Build history of the part. All positions in model axes, mm. Give positions to 0.01 mm unless a question says otherwise; leave off trailing zeros. Write each loop counter-clockwise with the first axis right and the second up, starting at its lowest first coordinate (ties: lowest second). Pieces come first, ordered by that corner, then holes. Notation, with made-up numbers: (23, 74.5) -> (50, 74.5) arc R33 cw to (50, 108.5) -> close; hole circle Ø7 at (33, -19). An arc over 180 degrees is marked (long way). Write item = value, one per line. Start each with the question number.
Q1. Saw through at C-C, the plane z = 0.3. Give the number of separate pieces and of enclosed holes in the cut face, then the cut area to 3 significant figures.
Q2. Wall check: line 1 (Y direction, x = 35, z = 1); line 2 (Y direction, x = 66, z = 1.05); line 3 (X direction, y = 85, z = 0.6). Give the ranges that are in metal, low to high.
Q3. Saw through at B-B, the plane x = 35. List the corners of the cut face in (y, z), then the cut area to 3 significant figures.
Q4. Saw through at A-A, the plane y = 75. List the corners of the cut face in (x, z).
Q5. Mould opens along X. For faces 1 (the face through (39.87, 121.66, 0.76)), 2 (the face through (40, 81, 0)) say: pulls with the +X half, pulls with the -X half, needs draft (parallel to the pull), parting line crosses it, or undercut.
from build123d import *

# Parameters (mm, degrees)
EXTRUDE_1_DEPTH      = 1.5
CUT_EXTRUDE_1_DEPTH  = 1.5
SKETCH_3_R           = 2
CUT_EXTRUDE_2_DEPTH  = 1.5
SKETCH_4_W           = 80
SKETCH_4_H           = 5
EXTRUDE_2_DEPTH      = 1.5
FILLET_1_R           = 2
SKETCH_5_OUTSIDE_W   = 163.618
SKETCH_5_OUTSIDE_H   = 213.618
SKETCH_5_OUTSIDE_W_2 = 80
SKETCH_5_OUTSIDE_H_2 = 170
CUT_EXTRUDE_3_DEPTH  = 193.943644622
SKETCH_6_R           = 1.5
CUT_EXTRUDE_4_DEPTH  = 184.377343202
SKETCH_7_W           = 6
SKETCH_7_H           = 170
CUT_EXTRUDE_5_DEPTH  = 10
FILLET_2_R           = 2
FILLET_3_R           = 1
FILLET_4_R           = 1


with BuildPart() as part:
    # 草图1 → 凸台-拉伸1 (new body)
    with BuildSketch(Plane.XY):
        Polygon((80, 90), (100, 90), (100, 70), (80, 70), (80, 0), (0, 0), (0, 70), (-20, 70), (-20, 90), (0, 90), (0, 160), (80, 160), align=None)
    extrude(amount=EXTRUDE_1_DEPTH)

    # 草图2 → 切除-拉伸1 (cut)
    with BuildSketch(Plane.XY.offset(1.5)):
        with BuildLine():
            Line((64, 153.5), (80, 153.5))
            Line((80, 153.5), (80, 156.5))
            Line((80, 156.5), (64, 156.5))
            ThreePointArc((64, 156.5), (62.5, 155), (64, 153.5))
        make_face()
        with BuildLine():
            Line((38.5, 5), (38.5, 15))
            ThreePointArc((38.5, 15), (40, 21.66227766), (41.5, 15))
            Line((41.5, 15), (41.5, 5))
            ThreePointArc((41.5, 5), (40, 3.5), (38.5, 5))
        make_face()
        with BuildLine():
            Line((16, 153.5), (0, 153.5))
            Line((0, 153.5), (0, 156.5))
            Line((0, 156.5), (16, 156.5))
            ThreePointArc((16, 156.5), (17.5, 155), (16, 153.5))
        make_face()
        with BuildLine():
            Line((64, 103.5), (80, 103.5))
            Line((80, 103.5), (80, 106.5))
            Line((80, 106.5), (64, 106.5))
            ThreePointArc((64, 106.5), (62.5, 105), (64, 103.5))
        make_face()
        with BuildLine():
            Line((16, 106.5), (0, 106.5))
            Line((0, 106.5), (0, 103.5))
            Line((0, 103.5), (16, 103.5))
            ThreePointArc((16, 103.5), (17.5, 105), (16, 106.5))
        make_face()
        with BuildLine():
            Line((16, 56.5), (0, 56.5))
            Line((0, 56.5), (0, 53.5))
            Line((0, 53.5), (16, 53.5))
            ThreePointArc((16, 53.5), (17.5, 55), (16, 56.5))
        make_face()
        with BuildLine():
            Line((64, 53.5), (80, 53.5))
            Line((80, 53.5), (80, 56.5))
            Line((80, 56.5), (64, 56.5))
            ThreePointArc((64, 56.5), (62.5, 55), (64, 53.5))
        make_face()
        with BuildLine():
            Line((16, 6.5), (0, 6.5))
            Line((0, 6.5), (0, 3.5))
            Line((0, 3.5), (16, 3.5))
            ThreePointArc((16, 3.5), (17.5, 5), (16, 6.5))
        make_face()
        with BuildLine():
            Line((64, 6.5), (80, 6.5))
            Line((80, 6.5), (80, 3.5))
            Line((80, 3.5), (64, 3.5))
            ThreePointArc((64, 3.5), (62.5, 5), (64, 6.5))
        make_face()
        with BuildLine():
            Line((38.5, 155), (38.5, 145))
            ThreePointArc((38.5, 145), (40, 138.33772234), (41.5, 145))
            Line((41.5, 145), (41.5, 155))
            ThreePointArc((41.5, 155), (40, 156.5), (38.5, 155))
        make_face()
        with BuildLine():
            Line((41.5, 55), (41.5, 45))
            ThreePointArc((41.5, 45), (40, 38.33772234), (38.5, 45))
            Line((38.5, 45), (38.5, 55))
            ThreePointArc((38.5, 55), (40, 56.5), (41.5, 55))
        make_face()
        with BuildLine():
            Line((38.5, 105), (38.5, 115))
            ThreePointArc((38.5, 115), (40, 121.66227766), (41.5, 115))
            Line((41.5, 115), (41.5, 105))
            ThreePointArc((41.5, 105), (40, 103.5), (38.5, 105))
        make_face()
    extrude(amount=-CUT_EXTRUDE_1_DEPTH, mode=Mode.SUBTRACT)

    # 草图3 → 切除-拉伸2 (cut)
    with BuildSketch(Plane.XY.offset(1.5)):
        with Locations((90, 80)):
            Circle(SKETCH_3_R)
        with Locations((-10, 80)):
            Circle(SKETCH_3_R)
    extrude(amount=-CUT_EXTRUDE_2_DEPTH, mode=Mode.SUBTRACT)

    # 草图4 → 凸台-拉伸2 (add)
    with BuildSketch(Plane(origin=(0, 0, 0), x_dir=(-1, 0, 0), z_dir=(0, 0, -1))):
        with Locations((-40, 162.5)):
            Rectangle(SKETCH_4_W, SKETCH_4_H)
        with Locations((-40, -2.5)):
            Rectangle(SKETCH_4_W, SKETCH_4_H)
    extrude(amount=-EXTRUDE_2_DEPTH)

    # 圆角1
    fillet_1_edges = [part.edges().sort_by_distance(p)[0] for p in [
        (0, 165, 0.75),
        (80, 165, 0.75),
        (0, -5, 0.75),
        (80, -5, 0.75),
    ]]
    fillet(fillet_1_edges, radius=FILLET_1_R)

    # 草图5 outside → 切除-拉伸3 (cut, through all)
    with BuildSketch(Plane.XY.offset(1.5)):
        with Locations((40, 80)):
            Rectangle(SKETCH_5_OUTSIDE_W, SKETCH_5_OUTSIDE_H)
        with Locations((40, 80)):
            Rectangle(SKETCH_5_OUTSIDE_W_2, SKETCH_5_OUTSIDE_H_2, mode=Mode.SUBTRACT)
    extrude(amount=-CUT_EXTRUDE_3_DEPTH, mode=Mode.SUBTRACT)

    # 草图6 → 切除-拉伸4 (cut, through all)
    with BuildSketch(Plane(origin=(0, 0, 0), x_dir=(-1, 0, 0), z_dir=(0, 0, -1))):
        with Locations((-35, 85)):
            Circle(SKETCH_6_R)
        with Locations((-35, 75)):
            Circle(SKETCH_6_R)
        with Locations(Location((-45, 75, 0), (0, 0, 180))):
            Circle(SKETCH_6_R)
        with Locations(Location((-45, 85, 0), (0, 0, 180))):
            Circle(SKETCH_6_R)
    extrude(amount=-CUT_EXTRUDE_4_DEPTH, mode=Mode.SUBTRACT)

    # 草图7 → 切除-拉伸5 (cut)
    with BuildSketch(Plane.XY.offset(1.5)):
        with Locations((3, 80)):
            Rectangle(SKETCH_7_W, SKETCH_7_H)
        with Locations((77, 80)):
            Rectangle(SKETCH_7_W, SKETCH_7_H)
    extrude(amount=-CUT_EXTRUDE_5_DEPTH, mode=Mode.SUBTRACT)

    # 圆角2
    fillet_2_edges = [part.edges().sort_by_distance(p)[0] for p in [
        (6, 165, 0.75),
        (6, -5, 0.75),
        (74, -5, 0.75),
        (74, 165, 0.75),
    ]]
    fillet(fillet_2_edges, radius=FILLET_2_R)

    # 圆角3
    fillet_3_edges = [part.edges().sort_by_distance(p)[0] for p in [
        (6, 156.5, 0.75),
        (6, 153.5, 0.75),
    ]]
    fillet(fillet_3_edges, radius=FILLET_3_R)

    # 圆角4
    fillet_4_edges = [part.edges().sort_by_distance(p)[0] for p in [
        (6, 106.5, 0.75),
        (6, 103.5, 0.75),
        (6, 56.5, 0.75),
        (6, 3.5, 0.75),
        (6, 53.5, 0.75),
        (6, 6.5, 0.75),
        (74, 156.5, 0.75),
        (74, 153.5, 0.75),
        (74, 106.5, 0.75),
        (74, 3.5, 0.75),
        (74, 103.5, 0.75),
        (74, 56.5, 0.75),
        (74, 6.5, 0.75),
        (74, 53.5, 0.75),
    ]]
    fillet(fillet_4_edges, radius=FILLET_4_R)


solid = part.part
Report:
q1.separate_pieces = 1
q1.enclosed_holes = 8
q1.area = 11,000 mm2
q2.line_1 = -5 to 73.5, 76.5 to 83.5, 86.5 to 165
q2.line_2 = -5 to 3.5, 6.5 to 53.5, 56.5 to 103.5, 106.5 to 153.5, 156.5 to 165
q2.line_3 = 6 to 33.5, 36.5 to 43.5, 46.5 to 74
q3.outline = (-5, 0) -> (73.5, 0) -> (73.5, 1.5) -> (-5, 1.5) -> close; (76.5, 0) -> (83.5, 0) -> (83.5, 1.5) -> (76.5, 1.5) -> close; (86.5, 0) -> (165, 0) -> (165, 1.5) -> (86.5, 1.5) -> close
q3.area = 246 mm2
q4.outline = (6, 0) -> (33.5, 0) -> (33.5, 1.5) -> (6, 1.5) -> close; (36.5, 0) -> (43.5, 0) -> (43.5, 1.5) -> (36.5, 1.5) -> close; (46.5, 0) -> (74, 0) -> (74, 1.5) -> (46.5, 1.5) -> close
q5.face_1 = undercut
q5.face_2 = needs draft
